Read the model definition and answer for the solid it produces. Units are mm, in the model's axes. A direction names the side the tool comes from. Give positions to 0.01 mm unless a question says otherwise; leave off trailing zeros. Loops run counter-clockwise (first coordinate to the right, second up) from the corner with the lowest first, then second, coordinate; pieces in that order, holes last. Notation, with made-up numbers: (-28.75, 27.25) - (-12.75, 27.25) arc R17 cw to (-12.75, 35.25) - close; hole circle Ø11 at (-38.5, -0.75). An arc over 180 degrees is marked (long way). Put each result on its own line as item: value. Start each with the question number.
1. For faces 1 (the cylindrical face through (-11.276, -14.154, 3.212)), 2 (the flat face through (5, -7, 9)), determine the directions among +Z, -Z, +X, -X, +Y, -Y from which every point of the face is accessible in a straight line to the end or side of a thin tool.
2. A cutting plane is placed at C-C, the plane z = 26.5. Determine the outline of the cut face in (x, y).
3. For a pull along Y with two mould halves and no side action, classify faces 3 (the cylindrical face through (-7.493, 0.33, 19.846)), 4 (the cylindrical face through (-0.822, -18.485, 3.212)), 5 (the flat face through (9.5, 5.2, 6)), 6 (the cylindrical face through (0.75, 5.7, 4.2)) as released by +Y, released by -Y, zero draft, split by the parting line, or undercut.
4. Consider L1, parallel to Y at x = 0, z = 5 (3 decimals); L2, parallel to X at y = 13, z = 3.5; L3, parallel to Z at x = 4.5, y = 3.5. Determine where each line is inside the solid, lowest interval first. Write a range as from..to.
5. Given pin 1 Ø10 at (x, y) = (-14.785, 0) entering from +Z; pin 2 Ø3 at (x, y) = (-1, -5) entering from -Z; pin 3 Ø1 at (x, y) = (11, 9) entering from +Z; pin 4 Ø3.5 at (x, y) = (-2.5, 1.5) entering from -Z, each flat-ended and moving along its own axis, determine where each tip first touches the part or whether it passes through.
6. A cutting plane is placed at A-A, the plane y = 0. Count the separate pieces of the cut face and the enclosed holes in it, plus the area to 3 significant figures.
```python
from build123d import *

# Parameters (mm, degrees)
SKETCH1_R           = 22
SKETCH1_R_2         = 3.79
SKETCH1_R_3         = 9
BOSS_EXTRUDE1_DEPTH = 6
SKETCH2_R           = 10.5
BOSS_EXTRUDE2_DEPTH = 25
SKETCH3_R           = 9
SKETCH3_R_2         = 5.75
BOSS_EXTRUDE3_DEPTH = 6
CHAMFER1_SIZE       = 0.5
CUT_EXTRUDE2_START  = -22
SKETCH4_R           = 10.5
SKETCH4_R_2         = 7.5
CUT_EXTRUDE2_DEPTH  = 22
SKETCH5_R           = 5.75
CUT_EXTRUDE3_DEPTH  = 8


with BuildPart() as part:
    # Sketch1 → Boss-Extrude1 (new body)
    with BuildSketch(Plane.XY):
        Circle(SKETCH1_R)
        with Locations((0, 14.785)):
            Circle(SKETCH1_R_2, mode=Mode.SUBTRACT)
        with Locations((10.45457376, 10.45457376)):
            Circle(SKETCH1_R_2, mode=Mode.SUBTRACT)
        with Locations((14.785, 0)):
            Circle(SKETCH1_R_2, mode=Mode.SUBTRACT)
        with Locations((10.45457376, -10.45457376)):
            Circle(SKETCH1_R_2, mode=Mode.SUBTRACT)
        with Locations((0, -14.785)):
            Circle(SKETCH1_R_2, mode=Mode.SUBTRACT)
        with Locations((-10.45457376, -10.45457376)):
            Circle(SKETCH1_R_2, mode=Mode.SUBTRACT)
        with Locations((-14.785, 0)):
            Circle(SKETCH1_R_2, mode=Mode.SUBTRACT)
        with Locations((-10.45457376, 10.45457376)):
            Circle(SKETCH1_R_2, mode=Mode.SUBTRACT)
        Circle(SKETCH1_R_3, mode=Mode.SUBTRACT)
    extrude(amount=BOSS_EXTRUDE1_DEPTH)

    # Sketch2 → Boss-Extrude2 (add)
    with BuildSketch(Plane.XY.offset(6)):
        Circle(SKETCH2_R)
    extrude(amount=BOSS_EXTRUDE2_DEPTH)

    # Sketch3 → Boss-Extrude3 (add)
    with BuildSketch(Plane(origin=(0, 0, 0), x_dir=(-1, 0, 0), z_dir=(0, 0, -1))):
        Circle(SKETCH3_R)
        Circle(SKETCH3_R_2, mode=Mode.SUBTRACT)
    extrude(amount=-BOSS_EXTRUDE3_DEPTH)

    # Chamfer1
    chamfer1_edges = [part.edges().sort_by_distance(p)[0] for p in [
        (6.66457376, 10.45457376, 0),
        (10.995, 0, 0),
        (-22, 0, 0),
        (6.66457376, -10.45457376, 0),
        (-3.79, -14.785, 0),
        (-14.24457376, -10.45457376, 0),
        (-18.575, 0, 0),
        (-14.24457376, 10.45457376, 0),
        (5.75, 0, 0),
        (-3.79, 14.785, 0),
    ]]
    chamfer(chamfer1_edges, length=CHAMFER1_SIZE)

    # Sketch4 → Cut-Extrude2 (cut)
    with BuildSketch(Plane.XY.offset(31).offset(CUT_EXTRUDE2_START)):
        Circle(SKETCH4_R)
        Circle(SKETCH4_R_2, mode=Mode.SUBTRACT)
    extrude(amount=CUT_EXTRUDE2_DEPTH, mode=Mode.SUBTRACT)

    # Sketch5 → Cut-Extrude3 (cut)
    with BuildSketch(Plane(origin=(0, 0, 0), x_dir=(-1, 0, 0), z_dir=(0, 0, -1))):
        Circle(SKETCH5_R)
    extrude(amount=-CUT_EXTRUDE3_DEPTH, mode=Mode.SUBTRACT)


solid = part.part
```
Return value:
1. face 1: +Z, -Z
1. face 2: +Z
2. outline: circle Ø15 at (0, 0)
3. face 3: split by the parting line
3. face 4: undercut
3. face 5: zero draft
3. face 6: undercut
4. L1: y = -22..-18.575, -10.995..-5.75, 5.75..10.995, 18.575..22
4. L2: x = -17.75..-13.26, -7.65..-3.34, 3.34..7.65, 13.26..17.75
4. L3: z = 8..31
5. pin 1: stops at z = 9
5. pin 2: stops at z = 0
5. pin 3: passes through
5. pin 4: stops at z = 8
6. separate pieces: 3
6. enclosed holes: 0
6. area: 473 mm2
